Design review of the part built by this model. Coordinates are the model's own, in mm. A direction names the side the tool comes from. Give positions to 0.01 mm unless a question says otherwise; leave off trailing zeros. Order: outer loops, then holes, each group sorted by start corner. A loop starts at its lowest first (then second) coordinate and runs counter-clockwise, first axis right, second up. Notation, with made-up numbers: (11.25, 81.5) -> (43.25, 81.5) arc R23 ccw to (43.25, 92.5) -> close; hole circle Ø10 at (7, -28). An arc over 180 degrees is marked (long way). Use a Markdown table: item, result. Add a question column.
Autodesk Inventor part; units mm, degrees
ref_plane "YZ Plane" through (0, 0, 0) normal (1, 0, 0) x (0, 1, 0)
ref_plane "XZ Plane" through (0, 0, 0) normal (0, 1, 0) x (-1, 0, 0)
ref_plane "XY Plane" through (0, 0, 0) normal (0, 0, 1) x (1, 0, 0)
sketch "Sketch3" plane through (0, 0, 0) normal (0, 1, 0) x (-1, 0, 0)
  circle A0 centre (11.1125, 0) radius 1.4906
  circle A1 centre (-5.5563, 9.6237) radius 1.4906
  circle A2 centre (-5.5562, -9.6237) radius 1.4906
  circle A3 centre (0, 0) radius 8.255
  line L0 (0, 0) -> (11.1125, 0)
  line L1 (0, 0) -> (-5.5563, 9.6237)
  line L2 (0, 0) -> (-5.5562, -9.6237)
  line L3 (0, 11.7306) -> (0, -34.9786)
  line L4 (38.6398, 0) -> (-3.2951, 0)
  circle A4 centre (40, 0) radius 5.05
  circle A5 centre (0, -40) radius 5.05
  circle A6 centre (0, 40) radius 5.05
  circle A7 centre (-40, 0) radius 5.05
  line L5 (-47.625, -47.625) -> (47.625, -47.625)
  line L6 (47.625, -47.625) -> (47.625, 47.625)
  line L7 (47.625, 47.625) -> (-47.625, 47.625)
  line L8 (-47.625, 47.625) -> (-47.625, -47.625)
  line L9 (-47.625, -47.625) -> (47.625, 47.625) construction
  line L10 (47.625, -47.625) -> (-47.625, 47.625) construction
  dimension "d19" = 120
  dimension "d20" = 120
  dimension "d21" = 11.1125
  dimension "d22" = 11.1125
  dimension "d23" = 11.1125
  dimension "d24" = 2.9811
  dimension "d25" = 2.9811
  dimension "d26" = 2.9811
  dimension "d27" = 80
  dimension "d28" = 80
  dimension "d29" = 10.1
  dimension "d30" = 10.1
  dimension "d31" = 95.25
  dimension "d32" = 95.25
  dimension "d36" = 16.51
extrude "Extrusion6" add sketch "Sketch3" along normal blind 6.35
fillet "Fillet1" radius 25.4 4 edges at (-47.625, 3.175, 47.625) (47.625, 3.175, 47.625) (47.625, 3.175, -47.625) (-47.625, 3.175, -47.625)
sketch "Sketch4" plane through (0, 6.35, 0) normal (0, 1, 0) x (1, 0, 0)
  line L0 (14.2748, 13.0048) -> (26.3652, 13.0048)
  line L1 (26.3652, 13.0048) -> (26.3652, -13.0048)
  line L2 (26.3652, -13.0048) -> (14.2748, -13.0048)
  line L3 (14.2748, -13.0048) -> (14.2748, 13.0048)
  line L4 (0, 0) -> (20.32, 0) construction
  point P0 (-11.2012, 0)
  point P1 (16.8026, 0)
  point P2 (26.3652, 0)
  point P3 (20.32, 13.0048)
  dimension "d39" = 12.0904
  dimension "d40" = 26.0096
  dimension "d41" = 20.32
extrude "Extrusion7" cut sketch "Sketch4" against normal up to next
fillet "Fillet2" radius 3.175 4 edges at (14.2748, 3.175, -13.0048) (14.2748, 3.175, 13.0048) (26.3652, 3.175, -13.0048) (26.3652, 3.175, 13.0048)
equation "\"d22\" = d21"
equation "\"d23\" = d21"
equation "\"d25\" = d24"
equation "\"d26\" = d24"
equation "\"d28\" = d27"
equation "\"d30\" = d29"
equation "\"d32\" = d31"
properties part number "Vertical_Lead_Screw_Plate_With_E-Stop"
1) Machinability: for faces 4 (the cylindrical face through (40.38, 3.22, -39.99)), 5 (the cylindrical face through (25.46, 3.13, 12.05)), which of the approach directions +Z, -Z, +X, -X, +Y, -Y give a long, thin tool a straight path to every point of the face, cutting with its end or side? Answer none if there is none.
2) For L1, parallel to Z at x = 0, y = 4.5 (3 decimals); L2, parallel to Z at x = 23, y = 2; L3, parallel to X at y = 1.25, z = -2.5 (3 decimals), list the stretches that pass through material, from the lowest coordinate up. Write a range as [from, to].
3) Add section C-C (y = 4.5). Give the number of separate pieces and of enclosed holes in the cut face, then the cut area to 3 significant figures.
4) The part is to be moulded in two halves that separate along X. For faces 1 (the flat face through (20, 3, -13.005)), 2 (the flat face through (1, 6.35, 11)), 3 (the cylindrical face through (-40.38, 3.22, 39.99)), say which applies: +X half, -X half, draft (parallel to the pull), parting line (faces both ways), or undercut.
5) Add section B-B (z = 0). Give the boundary of the cut face in (x, y) (3 decimals), then the cut area to 3 significant figures.
6) Add section A-A (x = 0). Give the boundary of the cut face in (y, z) (3 decimals), then the cut area to 3 significant figures.
7) Insertion check: pin 1 (1.5 mm diameter, centred on y = 2, z = -32.5, fed in from -X); pin 2 (2.5 mm diameter, centred on x = -11.11, z = 0, fed in from -Y); pin 3 (16 mm diameter, centred on x = 40, z = 0, fed in from -Y); pin 4 (1.5 mm diameter, centred on y = 5, z = -32.5, fed in from +X). Each pin has a flat end and moves straight along its axis. Give the tip position at first contact, or say it passes through.
8) Add section D-D (x = -40). Give the boundary of the cut face in (y, z), then the cut area to 3 significant figures.
Worked answers:
| question | item | result |
|---|---|---|
| 1 | face 4 | -Z, +X, +Y, -Y |
| 1 | face 5 | +Y, -Y |
| 2 | L1 | [-47.625, -45.05], [-34.95, -8.255], [8.255, 34.95], [45.05, 47.625] |
| 2 | L2 | [-47.61, -13], [13, 47.61] |
| 2 | L3 | [-47.625, -44.388], [-35.612, -7.867], [7.867, 14.275], [26.365, 35.612], [44.388, 47.625] |
| 3 | separate pieces | 1 |
| 3 | enclosed holes | 9 |
| 3 | area | 7,660 mm^2 |
| 4 | face 1 | undercut |
| 4 | face 2 | draft |
| 4 | face 3 | -X half |
| 5 | outline | (-47.625, 0) -> (-45.05, 0) -> (-45.05, 6.35) -> (-47.625, 6.35) -> close; (-34.95, 0) -> (-12.603, 0) -> (-12.603, 6.35) -> (-34.95, 6.35) -> close; (-9.622, 0) -> (-8.255, 0) -> (-8.255, 6.35) -> (-9.622, 6.35) -> close; (8.255, 0) -> (14.275, 0) -> (14.275, 6.35) -> (8.255, 6.35) -> close; (26.365, 0) -> (34.95, 0) -> (34.95, 6.35) -> (26.365, 6.35) -> close; (45.05, 0) -> (47.625, 0) -> (47.625, 6.35) -> (45.05, 6.35) -> close |
| 5 | area | 276 mm^2 |
| 6 | outline | (0, -47.625) -> (6.35, -47.625) -> (6.35, -45.05) -> (0, -45.05) -> close; (0, -34.95) -> (6.35, -34.95) -> (6.35, -8.255) -> (0, -8.255) -> close; (0, 8.255) -> (6.35, 8.255) -> (6.35, 34.95) -> (0, 34.95) -> close; (0, 45.05) -> (6.35, 45.05) -> (6.35, 47.625) -> (0, 47.625) -> close |
| 6 | area | 372 mm^2 |
| 7 | pin 1 | x = -45.77 |
| 7 | pin 2 | through |
| 7 | pin 3 | y = 0 |
| 7 | pin 4 | x = 45.77 |
| 8 | outline | (0, -40.37) -> (6.35, -40.37) -> (6.35, -5.05) -> (0, -5.05) -> close; (0, 5.05) -> (6.35, 5.05) -> (6.35, 40.37) -> (0, 40.37) -> close |
| 8 | area | 449 mm^2 |
